Can you work these out from the model? Positions are in its coordinate system, mm. A direction names the side the tool comes from. Give positions to 0.01 mm unless a question says otherwise; leave off trailing zeros. Loops run counter-clockwise (first coordinate to the right, second up) from the corner with the lowest first, then second, coordinate; pieces in that order, holes last. Notation, with made-up numbers: (33, -22.75) - (61, -22.75) arc R20 ccw to (61, -2.75) - close; hole circle Ø2 at (-1, 82.5). An arc over 180 degrees is marked (long way). Write item = value, one per line.
from build123d import *

# Parameters (mm, degrees)
SKETCH_1_W       = 23.45
SKETCH_1_H       = 62.3
EXTRUDE_1_DEPTH  = 2
SKETCH_2_W       = 5
SKETCH_2_H       = 5
SKETCH_2_H_2     = 8
EXTRUDE_2_DEPTH  = 1.5
CHAMFER_1_SIZE   = 1.5
CHAMFER_1_SIZE_2 = 7


with BuildPart() as part:
    # Эскиз1 → Бобышка-Вытянуть1 (new body)
    with BuildSketch(Plane.XY):
        with Locations((-11.445010077, -1532.80950355)):
            Rectangle(SKETCH_1_W, SKETCH_1_H)
    extrude(amount=EXTRUDE_1_DEPTH)

    # Эскиз2 → Бобышка-Вытянуть2 (add)
    with BuildSketch(Plane.XY.offset(2)):
        with Locations((-16.670010077, -1550.30950355)):
            Rectangle(SKETCH_2_W, SKETCH_2_H)
        with Locations((-6.220010077, -1532.80950355)):
            Rectangle(SKETCH_2_W, SKETCH_2_H_2)
        with Locations((-16.670010077, -1515.30950355)):
            Rectangle(SKETCH_2_W, SKETCH_2_H)
    extrude(amount=EXTRUDE_2_DEPTH)

    # Фаска1
    # the kernel refuses this chamfer: 7, 1.5 mm, written as the material it takes off along each edge
    with BuildSketch(Plane(origin=(-19.170010077, -1494.624450371, 3.5), x_dir=(-0.1730043027235695, 0, -0.9849210685324644), z_dir=(0, -1, 0))) as chamfer_1_piece_1_section:
        Polygon((CHAMFER_1_SIZE * 0.984921068532, CHAMFER_1_SIZE * 0.173004302724), (-CHAMFER_1_SIZE_2 * 0.173004302724, CHAMFER_1_SIZE_2 * 0.984921068532), (0, 0), align=None)
    chamfer_1_piece_1 = extrude(amount=41.370106359, mode=Mode.PRIVATE)
    chamfer_1_piece_1 = split(chamfer_1_piece_1, bisect_by=Plane(origin=(-16.689828283, -1515.30950355, 2), z_dir=(0, 0, 1)), keep=Keep.TOP, mode=Mode.PRIVATE)
    add(chamfer_1_piece_1, mode=Mode.SUBTRACT)
    with BuildSketch(Plane(origin=(-3.720010077, -1510.624450371, 3.5), x_dir=(0.17300430272357034, 0, -0.9849210685324644), z_dir=(0, -1, 0))) as chamfer_1_piece_2_section:
        Polygon((CHAMFER_1_SIZE * 0.984921068532, -CHAMFER_1_SIZE * 0.173004302724), (-CHAMFER_1_SIZE_2 * 0.173004302724, -CHAMFER_1_SIZE_2 * 0.984921068532), (0, 0), align=None)
    chamfer_1_piece_2 = extrude(amount=44.370106359, mode=Mode.PRIVATE)
    chamfer_1_piece_2 = split(chamfer_1_piece_2, bisect_by=Plane(origin=(-6.200191872, -1532.80950355, 2), z_dir=(0, 0, 1)), keep=Keep.TOP, mode=Mode.PRIVATE)
    add(chamfer_1_piece_2, mode=Mode.SUBTRACT)
    with BuildSketch(Plane(origin=(-19.170010077, -1529.624450371, 3.5), x_dir=(-0.1730043027235695, 0, -0.9849210685324644), z_dir=(0, -1, 0))) as chamfer_1_piece_3_section:
        Polygon((CHAMFER_1_SIZE * 0.984921068532, CHAMFER_1_SIZE * 0.173004302724), (-CHAMFER_1_SIZE_2 * 0.173004302724, CHAMFER_1_SIZE_2 * 0.984921068532), (0, 0), align=None)
    chamfer_1_piece_3 = extrude(amount=41.370106359, mode=Mode.PRIVATE)
    chamfer_1_piece_3 = split(chamfer_1_piece_3, bisect_by=Plane(origin=(-16.689828283, -1550.30950355, 2), z_dir=(0, 0, 1)), keep=Keep.TOP, mode=Mode.PRIVATE)
    add(chamfer_1_piece_3, mode=Mode.SUBTRACT)


solid = part.part
Q1. I need wall thicknesses on L1, parallel to Z at x = -18, y = -1519.5; L2, parallel to Z at x = -15.75, y = -1552. Which ranges of each line are inside material? Lowest first, please.
Output:
L1 = 0 to 2
L2 = 0 to 2.73
Q2. Which directions (+Z, -Z, +X, -X, +Y, -Y) give clear straight access to the entire face, cutting with the end or side of a thin tool? Please do faces 5 (the flat face through (-15.6, -1552.81, 2.3)), 6 (the flat face through (-6.8, -1528.81, 2.4)), 7 (the flat face through (-8.72, -1532.9, 2.5)), 8 (the flat face through (0.28, -1533, 1)), 9 (the flat face through (-14.17, -1550.3, 2.5)).
Output:
face_5 = +Z, +X, -X, -Y
face_6 = +Z, +X, -X, +Y
face_7 = +Z, -X, +Y, -Y
face_8 = +Z, -Z, +X, +Y, -Y
face_9 = +Z, +X, +Y, -Y
Q3. Imagine slicing it at D-D, the plane x = -11. Write out the boundary of the cut face in (y, z), then the cut area to 3 significant figures.
Output:
outline = (-1563.96, 0) - (-1501.66, 0) - (-1501.66, 2) - (-1563.96, 2) - close
area = 125 mm2
Q4. We'd pull the mould along Y, two halves only. Please class faces 1 (the flat face through (-23.17, -1533, 1)), 2 (the flat face through (-15.6, -1512.81, 2.3)), 3 (the flat face through (-15.6, -1517.81, 2.3)), 4 (the flat face through (-15.6, -1547.81, 2.3)): released by +Y, released by -Y, zero draft, split by the parting line, or undercut.
Output:
face_1 = zero draft
face_2 = released by +Y
face_3 = undercut
face_4 = undercut
Q5. Imagine slicing it at A-A, the plane y = -1516.5. Write out the boundary of the cut face in (x, z), then the cut area to 3 significant figures.
Output:
outline = (-23.17, 0) - (0.28, 0) - (0.28, 2) - (-14.17, 2) - (-14.17, 3.07) - (-19.17, 2) - (-23.17, 2) - close
area = 49.6 mm2
Q6. Imagine slicing it at B-B, the plane x = -15.25. Write out the boundary of the cut face in (y, z).
Output:
outline = (-1563.96, 0) - (-1501.66, 0) - (-1501.66, 2) - (-1512.81, 2) - (-1512.81, 2.84) - (-1517.81, 2.84) - (-1517.81, 2) - (-1547.81, 2) - (-1547.81, 2.84) - (-1552.81, 2.84) - (-1552.81, 2) - (-1563.96, 2) - close
Q7. Imagine slicing it at C-C, the plane x = -18.5. Write out the boundary of the cut face in (y, z).
Output:
outline = (-1563.96, 0) - (-1501.66, 0) - (-1501.66, 2) - (-1512.81, 2) - (-1512.81, 2.14) - (-1517.81, 2.14) - (-1517.81, 2) - (-1547.81, 2) - (-1547.81, 2.14) - (-1552.81, 2.14) - (-1552.81, 2) - (-1563.96, 2) - close
Q8. For pin 1 (11.5 mm diameter, centred on x = -13.5, y = -1542, fed in from +Z); pin 2 (0.9 mm diameter, centred on x = -15.5, z = 2.5, fed in from +Y); pin 3 (0.9 mm diameter, centred on y = -1515.5, z = 2.5, fed in from +X), each with a flat end and sliding along its axis, tell me the tip position at first contact or that it passes through.
Output:
pin_1 = 2
pin_2 = -1512.81
pin_3 = -14.17
